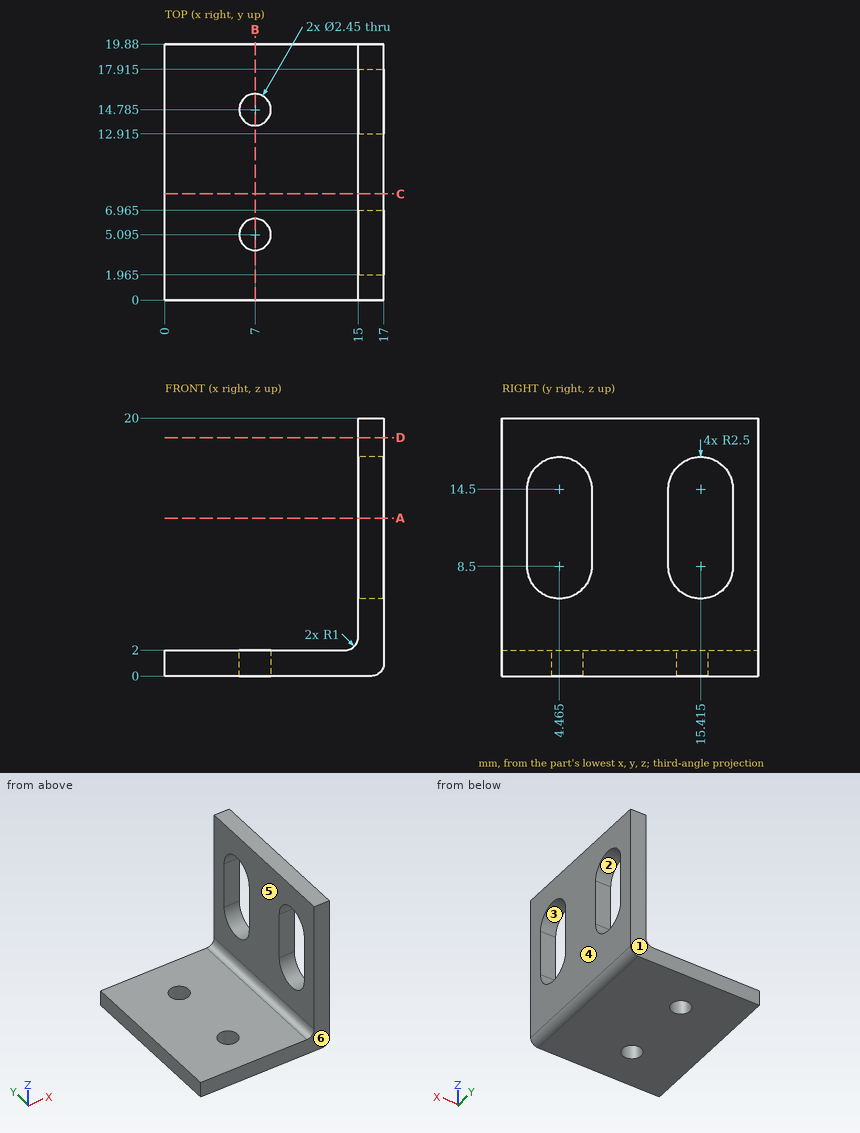
Here's the drawing with two shaded views (mm, measured from the low corner). I have some questions. A direction names the side the tool comes from. Coordinates: 2 decimals unless noted, no trailing zeros. Write each loop counter-clockwise with the first axis right and the second up, starting at its lowest first coordinate (ties: lowest second). Pieces come first, ordered by that corner, then holes. Notation, with made-up numbers: M 24.25,18 L 82.25,18 A29 ccw 82.25,49 Z; hole C 79.25,-6.5 d1. An arc over 180 degrees is marked long. Answer as CSV lines item,"result".
Item 1: Imagine slicing it at D-D on z = 18.5. List the corners of the cut face in (x, y) for me.
Geometry results:
outline,"M 15,0 L 17,0 L 17,19.88 L 15,19.88 Z"
Item 2: I'm going to push flat-ended pins straight in: P1, Ø4, axis at x = 4, y = 9, coming from the -Z side; P2, Ø3, axis at x = 7, y = 14.785, coming from the +Z side; P3, Ø5, axis at y = 6, z = 11, coming from the -X side. Where does each tip first touch, or does it pass through?
Geometry results:
P1,"stops at z = 0"
P2,"stops at z = 2"
P3,"stops at x = 15"
Item 3: Imagine slicing it at C-C on y = 8.25. List the corners of the cut face in (x, z) for me.
Geometry results:
outline,"M 0,0 L 16,0 A1 ccw 17,1 L 17,20 L 15,20 L 15,3 A1 cw 14,2 L 0,2 Z"
Item 4: Imagine slicing it at A-A on z = 12.25. List the corners of the cut face in (x, y) for me (1 decimal).
Geometry results:
outline,"M 15,0 L 17,0 L 17,2 L 15,2 Z; M 15,7 L 17,7 L 17,12.9 L 15,12.9 Z; M 15,17.9 L 17,17.9 L 17,19.9 L 15,19.9 Z"
Item 5: Imagine slicing it at B-B on x = 7. List the corners of the cut face in (y, z) for me.
Geometry results:
outline,"M 0,0 L 3.87,0 L 3.87,2 L 0,2 Z; M 6.32,0 L 13.56,0 L 13.56,2 L 6.32,2 Z; M 16.01,0 L 19.88,0 L 19.88,2 L 16.01,2 Z"
Item 6: On a 3-axis mill with a long thin cutter (end or side, diameter ignored), from which of +Z, -Z, +X, -X, +Y, -Y can I reach the whole of each face in a straight line? I mean the marked faces 5 and 6. Say none if no direction works.
Geometry results:
face 5,"+Z, -X, +Y, -Y"
face 6,"+Z, -Z, +X, -X, -Y"
Item 7: We'd pull the mould along Y, two halves only. Please class the marked faces 1, 2, 3 and 4: +Y half, -Y half, draft (parallel to the pull), parting line (faces both ways), or undercut.
Geometry results:
face 1,"+Y half"
face 2,"undercut"
face 3,"undercut"
face 4,"draft"
Item 8: Please list where these lines run through material, in increasing order: line 1 along Y through (x, z) = (7, 1.35); line 2 along X through (y, z) = (12.75, 12.5); line 3 along Z through (x, y) = (11.5, 13).
Geometry results:
line 1,"y = 0 to 3.87, 6.32 to 13.56, 16.01 to 19.88"
line 2,"x = 15 to 17"
line 3,"z = 0 to 2"
